```python
from build123d import *

# Parameters (mm, degrees)
SKETCH1_R           = 30
BOSS_EXTRUDE1_DEPTH = 5
SKETCH2_R           = 19.5
BOSS_EXTRUDE2_DEPTH = 1
SKETCH3_R           = 17.5
BOSS_EXTRUDE3_DEPTH = 15
SKETCH4_R           = 12.025
CUT_EXTRUDE1_DEPTH  = 7
SKETCH5_R           = 10.5
CUT_EXTRUDE2_DEPTH  = 45.676615807
SKETCH6_R           = 1.75
CUT_EXTRUDE3_DEPTH  = 46.343136195
SKETCH7_R           = 1.75
CUT_EXTRUDE4_DEPTH  = 10
SKETCH8_R           = 1.225
CUT_EXTRUDE5_DEPTH  = 12
CUT_EXTRUDE6_DEPTH  = 3.25


with BuildPart() as part:
    # Sketch1 → Boss-Extrude1 (new body)
    with BuildSketch(Plane.XY):
        Circle(SKETCH1_R)
    extrude(amount=BOSS_EXTRUDE1_DEPTH)

    # Sketch2 → Boss-Extrude2 (add)
    with BuildSketch(Plane.XY.offset(5)):
        Circle(SKETCH2_R)
    extrude(amount=BOSS_EXTRUDE2_DEPTH)

    # Sketch3 → Boss-Extrude3 (add)
    with BuildSketch(Plane.XY.offset(6)):
        Circle(SKETCH3_R)
    extrude(amount=BOSS_EXTRUDE3_DEPTH)

    # Sketch4 → Cut-Extrude1 (cut)
    with BuildSketch(Plane(origin=(0, 0, 0), x_dir=(-1, 0, 0), z_dir=(0, 0, -1))):
        Circle(SKETCH4_R)
    extrude(amount=-CUT_EXTRUDE1_DEPTH, mode=Mode.SUBTRACT)

    # Sketch5 → Cut-Extrude2 (cut, through all)
    with BuildSketch(Plane(origin=(0, 0, 7), x_dir=(-1, 0, 0), z_dir=(0, 0, -1))):
        Circle(SKETCH5_R)
    extrude(amount=-CUT_EXTRUDE2_DEPTH, mode=Mode.SUBTRACT)

    # Sketch6 → Cut-Extrude3 (cut, through all)
    with BuildSketch(Plane.XY.offset(5)):
        with Locations((24.5, 0)):
            Circle(SKETCH6_R)
        with Locations((12.25, -21.217622393)):
            Circle(SKETCH6_R)
        with Locations((-12.25, -21.217622393)):
            Circle(SKETCH6_R)
        with Locations((-24.5, 0)):
            Circle(SKETCH6_R)
        with Locations((-12.25, 21.217622393)):
            Circle(SKETCH6_R)
        with Locations((12.25, 21.217622393)):
            Circle(SKETCH6_R)
    extrude(amount=-CUT_EXTRUDE3_DEPTH, mode=Mode.SUBTRACT)

    # Sketch7 → Cut-Extrude4 (cut)
    with BuildSketch(Plane.XY.offset(21)):
        with Locations((14, 0)):
            Circle(SKETCH7_R)
        with Locations((7, -12.124355653)):
            Circle(SKETCH7_R)
        with Locations((-7, -12.124355653)):
            Circle(SKETCH7_R)
        with Locations((-14, 0)):
            Circle(SKETCH7_R)
        with Locations((-7, 12.124355653)):
            Circle(SKETCH7_R)
        with Locations((7, 12.124355653)):
            Circle(SKETCH7_R)
    extrude(amount=-CUT_EXTRUDE4_DEPTH, mode=Mode.SUBTRACT)

    # Sketch8 → Cut-Extrude5 (cut)
    with BuildSketch(Plane.XY.offset(21)):
        with Locations((12.124355653, 7)):
            Circle(SKETCH8_R)
        with Locations((0, -14)):
            Circle(SKETCH8_R)
        with Locations((-12.124355653, 7)):
            Circle(SKETCH8_R)
    extrude(amount=-CUT_EXTRUDE5_DEPTH, mode=Mode.SUBTRACT)

    # Sketch9 → Cut-Extrude6 (cut)
    with BuildSketch(Plane.XY.offset(5)):
        Polygon((12.25, -16.967622393), (8.569392034, -19.092622393), (8.569392034, -23.342622393), (12.25, -25.467622393), (15.930607966, -23.342622393), (15.930607966, -19.092622393), align=None)
        Polygon((24.5, 4.25), (20.819392034, 2.125), (20.819392034, -2.125), (24.5, -4.25), (28.180607966, -2.125), (28.180607966, 2.125), align=None)
        Polygon((-8.569392034, -19.092622393), (-12.25, -16.967622393), (-15.930607966, -19.092622393), (-15.930607966, -23.342622393), (-12.25, -25.467622393), (-8.569392034, -23.342622393), align=None)
        Polygon((-20.819392034, -2.125), (-20.819392034, 2.125), (-24.5, 4.25), (-28.180607966, 2.125), (-28.180607966, -2.125), (-24.5, -4.25), align=None)
        Polygon((-12.25, 16.967622393), (-8.569392034, 19.092622393), (-8.569392034, 23.342622393), (-12.25, 25.467622393), (-15.930607966, 23.342622393), (-15.930607966, 19.092622393), align=None)
        Polygon((8.569392034, 19.092622393), (12.25, 16.967622393), (15.930607966, 19.092622393), (15.930607966, 23.342622393), (12.25, 25.467622393), (8.569392034, 23.342622393), align=None)
    extrude(amount=-CUT_EXTRUDE6_DEPTH, mode=Mode.SUBTRACT)


solid = part.part
```
CAD build for the part. Positions are in the model's coordinates, mm. A direction names the side the tool comes from. Coordinates: 2 decimals unless noted, no trailing zeros. Loops run counter-clockwise (first coordinate to the right, second up) from the corner with the lowest first, then second, coordinate; pieces in that order, holes last. Notation, with made-up numbers: (34, 39.25) - (69, 39.25) arc R19 ccw to (69, 65.25) - close; hole circle Ø6 at (-26, -19.5). An arc over 180 degrees is marked (long way). Use CSV: the item, a comma, the result in double quotes. Start each with the question number.
Q1. Two-plate mould, pull along Y, no slides. Class faces 3 (the flat face through (22.685, 3.202, 3.398)), 4 (the cylindrical face through (-29.97, 1.32, 2.46)), 5 (the flat face through (-10.4, 24.4, 3.4)): +Y half, -Y half, draft (parallel to the pull), parting line (faces both ways), or undercut.
Q2. Probe probe 1 along Y at (x, z) = (0, 18.75) (3 decimals); probe 2 along Y at (x, z) = (-10.5, 2.75); probe 3 along X at (y, z) = (-23, 3.75). List the from-to ranges inside material, lowest first. Write a range as from..to.
Q3. Cut at C-C, the plane y = 22. List the corners of the cut face in (x, z).
Q4. Drop flat-ended pins along their axis: P1, Ø2.5, axis at y = -20.5, z = 3, coming from the -X side; P2, Ø3.5, axis at y = -22, z = 3.5, coming from the +X side; P3, Ø8, axis at x = -11.5, y = 23, coming from the +Z side; P4, Ø6, axis at x = 0.5, y = 6, coming from the -Z side. Give the stop position or say it passes through.
Q5. Cut at A-A, the plane y = 5. List the corners of the cut face in (x, z), then the cut area to 3 significant figures.
Q6. 3-axis set-ups, long thin cutter, end or side, ignore diameter. For faces 1 (the cylindrical face through (-26.25, 0.08, 0.89)), 2 (the flat face through (-14, -22, 1.75)): which of +Z, -Z, +X, -X, +Y, -Y reach the whole face in a straight line?
Q7. Cut at D-D, the plane z = 16. State how many separate pieces and enclosed holes the cut face has, then the cut area to 3 significant figures.
Q8. Cut at B-B, the plane x = 4.5. List the corners of the cut face in (y, z).
Here are the results:
1,face 3,"undercut"
1,face 4,"parting line"
1,face 5,"undercut"
2,probe 1,"-17.5..-15.225, -12.775..-10.5, 10.5..17.5"
2,probe 2,"-28.1..-24.46, -17.98..-5.86, 5.86..17.98, 24.46..28.1"
2,probe 3,"-19.26..-15.93, -8.57..8.57, 15.93..19.26"
3,outline,"(-20.4, 0) - (-13.82, 0) - (-13.82, 1.75) - (-15.93, 1.75) - (-15.93, 5) - (-20.4, 5) - close; (-10.68, 0) - (10.68, 0) - (10.68, 1.75) - (8.57, 1.75) - (8.57, 5) - (-8.57, 5) - (-8.57, 1.75) - (-10.68, 1.75) - close; (13.82, 0) - (20.4, 0) - (20.4, 5) - (15.93, 5) - (15.93, 1.75) - (13.82, 1.75) - close"
4,P1,"x = -23.01"
4,P2,"x = 22.13"
4,P3,"z = 5"
4,P4,"through"
5,outline,"(-29.58, 0) - (-10.94, 0) - (-10.94, 7) - (-9.23, 7) - (-9.23, 21) - (-16.77, 21) - (-16.77, 6) - (-18.85, 6) - (-18.85, 5) - (-29.58, 5) - close; (9.23, 7) - (10.94, 7) - (10.94, 0) - (29.58, 0) - (29.58, 5) - (18.85, 5) - (18.85, 6) - (16.77, 6) - (16.77, 21) - (9.23, 21) - close"
5,area,"425 mm2"
6,face 1,"+Z, -Z"
6,face 2,"+Z"
7,separate pieces,"1"
7,enclosed holes,"10"
7,area,"544 mm2"
8,outline,"(-29.66, 0) - (-11.15, 0) - (-11.15, 7) - (-9.49, 7) - (-9.49, 21) - (-16.91, 21) - (-16.91, 6) - (-18.97, 6) - (-18.97, 5) - (-29.66, 5) - close; (9.49, 7) - (11.15, 7) - (11.15, 0) - (29.66, 0) - (29.66, 5) - (18.97, 5) - (18.97, 6) - (16.91, 6) - (16.91, 21) - (9.49, 21) - close"
